```python
from build123d import *

# Parameters (mm, degrees)
SKETCH1_W           = 5
SKETCH1_H           = 70
SKETCH1_W_2         = 70
SKETCH1_H_2         = 60
BOSS_EXTRUDE1_DEPTH = 35
SKETCH2_R           = 21
CUT_EXTRUDE1_DEPTH  = 127.984250992
CHAMFER1_SIZE       = 4
CHAMFER2_SIZE       = 4
SKETCH9_W           = 10
SKETCH9_H           = 20
BOSS_EXTRUDE2_DEPTH = 70
RIB1_REACH          = 128.984
SKETCH10_WALL_W     = 330.29884572
SKETCH10_WALL_H     = 4
SKETCH11_W          = 5
SKETCH11_H          = 5
CUT_EXTRUDE2_DEPTH  = 10


with BuildPart() as part:
    # Sketch1 → Boss-Extrude1 (new, symmetric)
    with BuildSketch(Plane(origin=(0, 0, 0), x_dir=(0, 0, -1), z_dir=(1, 0, 0))):
        with Locations((-32.5, 65)):
            Rectangle(SKETCH1_W, SKETCH1_H)
        Rectangle(SKETCH1_W_2, SKETCH1_H_2)
    extrude(amount=BOSS_EXTRUDE1_DEPTH, both=True)

    # Sketch2 → Cut-Extrude1 (cut, through all)
    with BuildSketch(Plane(origin=(0, 0, -35), x_dir=(-1, 0, 0), z_dir=(0, 0, -1))):
        Circle(SKETCH2_R)
    extrude(amount=-CUT_EXTRUDE1_DEPTH, mode=Mode.SUBTRACT)

    # Chamfer1
    chamfer1_edges = [part.edges().sort_by_distance(p)[0] for p in [
        (21, 0, 35),
    ]]
    chamfer(chamfer1_edges, length=CHAMFER1_SIZE)

    # Chamfer2
    chamfer2_edges = [part.edges().sort_by_distance(p)[0] for p in [
        (21, 0, -35),
    ]]
    chamfer(chamfer2_edges, length=CHAMFER2_SIZE)

    # Sketch9 → Boss-Extrude2 (add, through all)
    with BuildSketch(Plane(origin=(35, 0, 0), x_dir=(0, 0, -1), z_dir=(1, 0, 0))):
        with Locations((-25, 90)):
            Rectangle(SKETCH9_W, SKETCH9_H)
    extrude(amount=-BOSS_EXTRUDE2_DEPTH)

    # Sketch10 wall → Rib1 (add, up to next)
    with BuildSketch(Plane(origin=(35, 55, -7.5), x_dir=(0, -0.672672793996, -0.739940073396), z_dir=(0, 0.739940073396, -0.672672793996)), mode=Mode.PRIVATE) as rib1_sk1:
        with Locations((0, 2)):
            Rectangle(SKETCH10_WALL_W, SKETCH10_WALL_H)
    rib1_tool1 = extrude(rib1_sk1.sketch, amount=-RIB1_REACH, mode=Mode.PRIVATE) - part.part
    rib1 = rib1_tool1.solids().sort_by_distance((35, 55, -7.5))[0]
    add(rib1)

    # Mirror1: Rib1 across plane
    add(rib1.mirror(Plane(origin=(0, 0, 0), x_dir=(0, 0, 1), z_dir=(1, 0, 0))))

    # Sketch11 → Cut-Extrude2 (cut)
    with BuildSketch(Plane.XY.offset(35)):
        with Locations((15, 91.5)):
            Rectangle(SKETCH11_W, SKETCH11_H)
        with Locations((-15, 91.5)):
            Rectangle(SKETCH11_W, SKETCH11_H)
    extrude(amount=-CUT_EXTRUDE2_DEPTH, mode=Mode.SUBTRACT)


solid = part.part
```
Could you check a few things on this model? Use its own coordinates, in mm. A direction names the side the tool comes from. Give positions to 0.01 mm unless a question says otherwise; leave off trailing zeros. Loops run counter-clockwise (first coordinate to the right, second up) from the corner with the lowest first, then second, coordinate; pieces in that order, holes last. Notation, with made-up numbers: (2.25, -8.5) - (13.25, -8.5) arc R17 ccw to (13.25, 21.5) - close; hole circle Ø7 at (41, 17). An arc over 180 degrees is marked (long way). Use one line per item in the form item = value.
1. I want a section at D-D (z = 23.5). Please give me the cut outline in (x, y).
Response values:
outline = (-35, -30) - (35, -30) - (35, 100) - (-35, 100) - close; hole (-31, 30) - (31, 30) - (31, 80) - (-31, 80) - close; hole circle Ø42 at (0, 0)
2. Thinking about a two-plate mould opening in X: for faces 1 (the face through (0, 100, 28)), 2 (the face through (12.5, 91, 30)), which applies, released by +X, released by -X, zero draft, split by the parting line, or undercut?
Response values:
face_1 = zero draft
face_2 = undercut
3. I want a section at A-A (x = 0). Please give me the cut outline in (y, z), and give its area (3 significant figures).
Response values:
outline = (-30, -35) - (-25, -35) - (-21, -31) - (-21, 31) - (-25, 35) - (-30, 35) - close; (21, -31) - (25, -35) - (30, -35) - (30, 30) - (80, 30) - (80, 20) - (100, 20) - (100, 35) - (25, 35) - (21, 31) - close
area = 1,780 mm²
4. I want a section at B-B (z = -29.5). Please give me the cut outline in (x, y), and give its area (3 significant figures).
Response values:
outline = (-35, -30) - (35, -30) - (35, 35) - (31, 35) - (31, 30) - (-31, 30) - (-31, 35) - (-35, 35) - close; hole circle Ø42 at (0, 0)
area = 2,850 mm²
5. On a 3-axis mill with a long thin cutter (end or side, diameter ignored), from which of +Z, -Z, +X, -X, +Y, -Y can I reach the whole of each face in a straight line? I mean faces 3 (the face through (16, -20, -35)), 4 (the face through (-31, 46, 7)), 5 (the face through (-12.5, 91, 30)). Say none if no direction works.
Response values:
face_3 = -Z, +X, -X, +Y, -Y
face_4 = -Z
face_5 = +Z
6. I'm going to push flat-ended pins straight in: pin 1 Ø12 at (x, z) = (22.5, -10) entering from +Y; pin 2 Ø10 at (x, y) = (7, 94.5) entering from -Z; pin 3 Ø2.5 at (x, y) = (14, 92.5) entering from +Z. Where does each tip first touch, or does it pass through?
Response values:
pin_1 = 30
pin_2 = 20
pin_3 = 25
7. I want a section at C-C (y = 0). Please give me the cut outline in (x, z).
Response values:
outline = (-35, -35) - (-25, -35) - (-21, -31) - (-21, 31) - (-25, 35) - (-35, 35) - close; (21, -31) - (25, -35) - (35, -35) - (35, 35) - (25, 35) - (21, 31) - close
8. I need wall thicknesses on probe 1 along X at (y, z) = (36.5, -25); probe 2 along Y at (x, z) = (0, 5); probe 3 along Y at (x, z) = (8, 24). Which ranges of each line are inside material? Lowest first, please.
Response values:
probe_1 = -35 to -31, 31 to 35
probe_2 = -30 to -21, 21 to 30
probe_3 = -30 to -19.42, 19.42 to 30, 80 to 100
